Geometry check sheet. Reference: drawing and pictorial views, mm from the part's lowest x, y, z. A direction names the side the tool comes from. Round coordinates to 2 decimals unless told otherwise and drop trailing zeros. Order: outer loops, then holes, each group sorted by start corner. A loop starts at its lowest first (then second) coordinate and runs counter-clockwise, first axis right, second up.
Q1. Cross-section at D-D on x = 5.5. Record the cut outline in (y, z) (3 decimals).
Q2. Cross-section at C-C on z = 32. Record the cut outline in (x, y).
Q3. Depth check by flat-ended pin: P1, Ø5, axis at x = 5, z = 5, coming from the +Y side; P2, Ø1, axis at x = 14, z = 19, coming from the +Y side; P3, Ø12, axis at x = 14, y = 18, coming from the +Z side; P4, Ø3, axis at x = 16.5, z = 11.5, coming from the -Y side. Enter the tip coordinate at first touch or a pass-through.
Q4. Set-up check for the marked faces 1 and 2: record each of +Z, -Z, +X, -X, +Y, -Y from which the full face is reachable in a straight line by a thin tool's end or side.
Q5. Scan lines: probe 1 along X at (y, z) = (10.5, 31.5); probe 2 along Z at (x, y) = (17.25, 6.5). Record each from-to range of solid material in increasing order.
Q6. Cross-section at A-A on x = 10.5. Record the cut outline in (y, z).
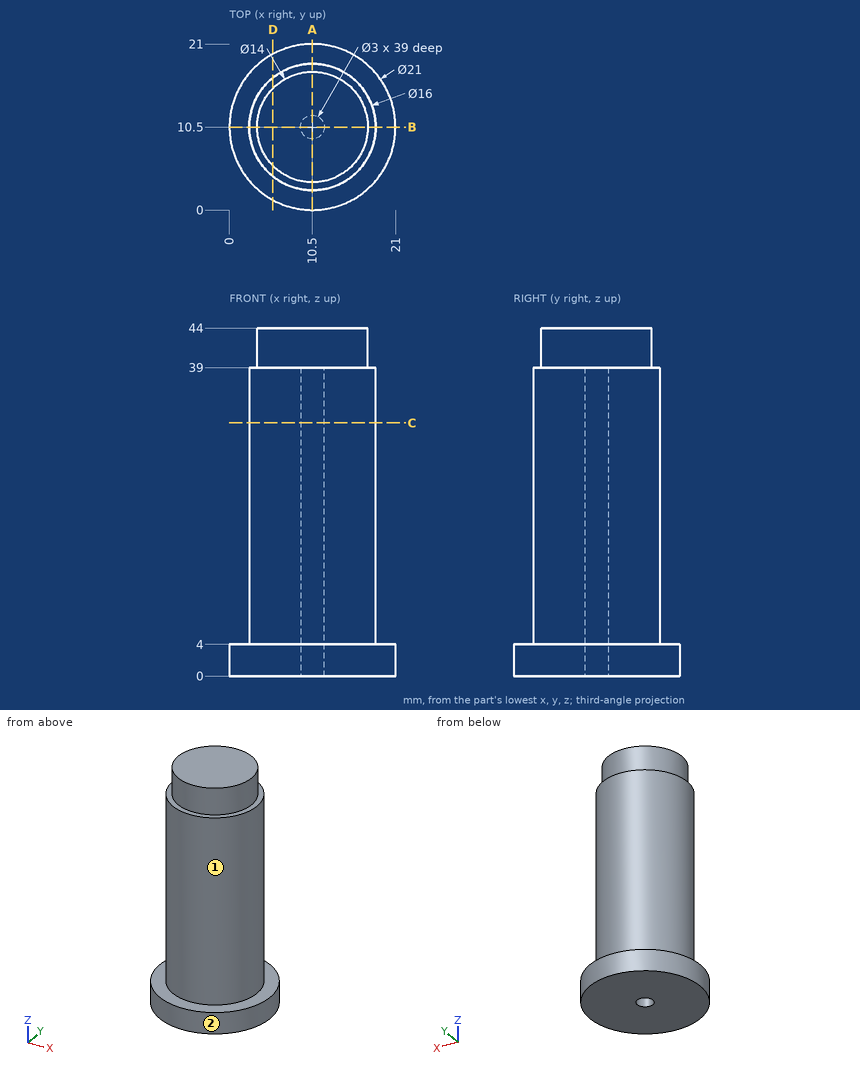
Results found:
1. outline: (1.267, 0) - (19.733, 0) - (19.733, 4) - (16.745, 4) - (16.745, 39) - (15.399, 39) - (15.399, 44) - (5.601, 44) - (5.601, 39) - (4.255, 39) - (4.255, 4) - (1.267, 4) - close
2. outline: circle Ø16 at (10.5, 10.5); hole circle Ø3 at (10.5, 10.5)
3. P1: stops at y = 20.5
3. P2: stops at y = 17.92
3. P3: stops at z = 44
3. P4: stops at y = 3.89
4. face 1: +Z
4. face 2: +Z, -Z
5. probe 1: x = 2.5 to 9, 12 to 18.5
5. probe 2: z = 0 to 39
6. outline: (0, 0) - (9, 0) - (9, 39) - (12, 39) - (12, 0) - (21, 0) - (21, 4) - (18.5, 4) - (18.5, 39) - (17.5, 39) - (17.5, 44) - (3.5, 44) - (3.5, 39) - (2.5, 39) - (2.5, 4) - (0, 4) - close
